Input: part model. Units: mm. Frame: model coordinates. A direction names the side the tool comes from. Round coordinates to 2 decimals unless told otherwise and drop trailing zeros. Order: outer loops, then holes, each group sorted by start corner. A loop starts at its lowest first (then second) coordinate and runs counter-clockwise, first axis right, second up. Notation, with made-up numbers: M -40,28.25 L -32,28.25 A20 ccw -32,38.25 Z; hole C 72,53.25 d4. An arc over 180 degrees is marked long. One line per question, with ' | ' between items.
```python
from build123d import *

# Parameters (mm, degrees)
SKETCH1_R             = 7
BOSS_EXTRUDE1_DEPTH   = 30
BOSS_EXTRUDE2_START   = -25
SKETCH3_R             = 7
SKETCH3_R_2           = 4.25
BOSS_EXTRUDE2_DEPTH   = 20
F_2_0MM_DOWEL_HOLE1_D = 2


with BuildPart() as part:
    # Sketch1 → Boss-Extrude1 (new body)
    # profile 1 of 2: a face of its own
    with BuildSketch(Plane.XY):
        Polygon((-16.25, 6.5), (16.25, 6.5), (16.25, -4.427166083), (17.25, -5.5), (17.25, -10.5), (8.5, -10.5), (8, -10), (-8, -10), (-8.5, -10.5), (-9, -10.5), (-17.25, -10.5), (-17.25, -5.5), (-16.25, -4.427166083), align=None)
        with Locations((0, 0.5)):
            Circle(SKETCH1_R, mode=Mode.SUBTRACT)
    # profile 2 of 2: a face of its own
    with BuildSketch(Plane.XY):
        with BuildLine():
            Line((3.605551275, 6.5), (8.25, 6.5))
            Line((8.25, 6.5), (4.25, 10.5))
            Line((4.25, 10.5), (-5.25, 10.5))
            Line((-5.25, 10.5), (-9.25, 6.5))
            Line((-9.25, 6.5), (-3.605551275, 6.5))
            ThreePointArc((-3.605551275, 6.5), (0, 7.5), (3.605551275, 6.5))
        make_face()
    extrude(amount=BOSS_EXTRUDE1_DEPTH)

    # Sketch3 → Boss-Extrude2 (add)
    with BuildSketch(Plane.XY.offset(30).offset(BOSS_EXTRUDE2_START)):
        with Locations((0, 0.5)):
            Circle(SKETCH3_R)
        with Locations((0, 0.5)):
            Circle(SKETCH3_R_2, mode=Mode.SUBTRACT)
    extrude(amount=BOSS_EXTRUDE2_DEPTH)

    # Ø2.0mm Dowel Hole1 (through all)
    with Locations(Plane(origin=(0, -10.5, 0), x_dir=(-1, 0, 0), z_dir=(0, -1, 0))):
        with Locations((11.5, -25), (11.5, -5), (-11.5, -5), (-11.5, -25)):
            Hole(F_2_0MM_DOWEL_HOLE1_D / 2)


solid = part.part
```
Item 1: First-contact query: pin 1 (2.5 mm diameter, centred on x = -11.5, z = 5, fed in from +Y); pin 2 (7 mm diameter, centred on x = -2, y = 2.5, fed in from +Z); pin 3 (12 mm diameter, centred on y = 1, z = 16.5, fed in from -X). Flat tips, straight axial feed; report the tip coordinate or a pass-through.
Report:
pin 1: y = 6.5 | pin 2: z = 25 | pin 3: x = -16.78
Item 2: Section query B-B, the plane x = -11.5. Return loops of the section in (y, z).
Report:
outline: M -10.5,0 L 6.5,0 L 6.5,4 L -10.5,4 Z; M -10.5,6 L 6.5,6 L 6.5,24 L -10.5,24 Z; M -10.5,26 L 6.5,26 L 6.5,30 L -10.5,30 Z
Item 3: Line query: line 1 along Z through (x, y) = (-11.5, -5.75); line 2 along Y through (x, z) = (0, 15.25); line 3 along Y through (x, z) = (10, 13.5). Output: solid intervals per line, ascending. Write a range as from..to.
Report:
line 1: 0..4, 6..24, 26..30 | line 2: -10..-3.75, 4.75..10.5 | line 3: -10.5..6.5
Item 4: Mould query, pull axis X, two halves, no side actions, for faces 6 (the flat face through (6.28, 8.47, 14.79)), 7 (the flat face through (3, -3, 25)), 8 (the flat face through (0, -7, 30)). Classes: +X half, -X half, draft (parallel to the pull), parting line (faces both ways), or undercut.
Report:
face 6: +X half | face 7: undercut | face 8: draft
Item 5: Section query C-C, the plane z = 16.25. Return loops of the section in (x, y), plus the area to 3 significant figures.
Report:
outline: M -17.25,-10.5 L -8.5,-10.5 L -8,-10 L 8,-10 L 8.5,-10.5 L 17.25,-10.5 L 17.25,-5.5 L 16.25,-4.43 L 16.25,6.5 L 8.25,6.5 L 4.25,10.5 L -5.25,10.5 L -9.25,6.5 L -16.25,6.5 L -16.25,-4.43 L -17.25,-5.5 Z; hole C 0,0.5 d8.5 | area: 553 mm²
Item 6: Section query A-A, the plane y = 0.5. Return loops of the section in (x, z).
Report:
outline: M -16.25,0 L -7,0 L -7,5 L -4.25,5 L -4.25,25 L -7,25 L -7,30 L -16.25,30 Z; M 4.25,5 L 7,5 L 7,0 L 16.25,0 L 16.25,30 L 7,30 L 7,25 L 4.25,25 Z; hole C -11.5,5 d2; hole C -11.5,25 d2; hole C 11.5,5 d2; hole C 11.5,25 d2
Item 7: Section query D-D, the plane x = 2. Return loops of the section in (y, z).
Report:
outline: M -10,0 L -6.21,0 L -6.21,5 L -3.25,5 L -3.25,25 L -6.21,25 L -6.21,30 L -10,30 Z; M 4.25,5 L 7.21,5 L 7.21,0 L 10.5,0 L 10.5,30 L 7.21,30 L 7.21,25 L 4.25,25 Z
Item 8: Access query for faces 1 (the flat face through (3, -3, 5)), 2 (the flat face through (0, 10.5, 15)), 3 (the flat face through (-13, 6.5, 15)), 4 (the flat face through (16.25, 1, 15)), 5 (the flat face through (0, -10, 15)). Directions: +Z, -Z, +X, -X, +Y, -Y. A direction counts if a zero-diameter tool reaches every point of the face in a straight line with its end or side. Return the directions, or none.
Report:
face 1: -Z | face 2: +Z, -Z, +X, -X, +Y | face 3: +Z, -Z, -X, +Y | face 4: +Z, -Z, +X, +Y | face 5: +Z, -Z, -Y
